Part print with two shaded views. Sizes in mm from the minimum x, y, z corner. Round coordinates to 2 decimals unless told otherwise and drop trailing zeros. Write each loop counter-clockwise with the first axis right and the second up, starting at its lowest first coordinate (ties: lowest second). Pieces come first, ordered by that corner, then holes. Notation, with made-up numbers: (2, 81) -> (57, 81) arc R22 ccw to (57, 106) -> close; hole circle Ø10 at (-23, -13). An arc over 180 degrees is marked (long way). Answer in a Markdown table with one row per item.
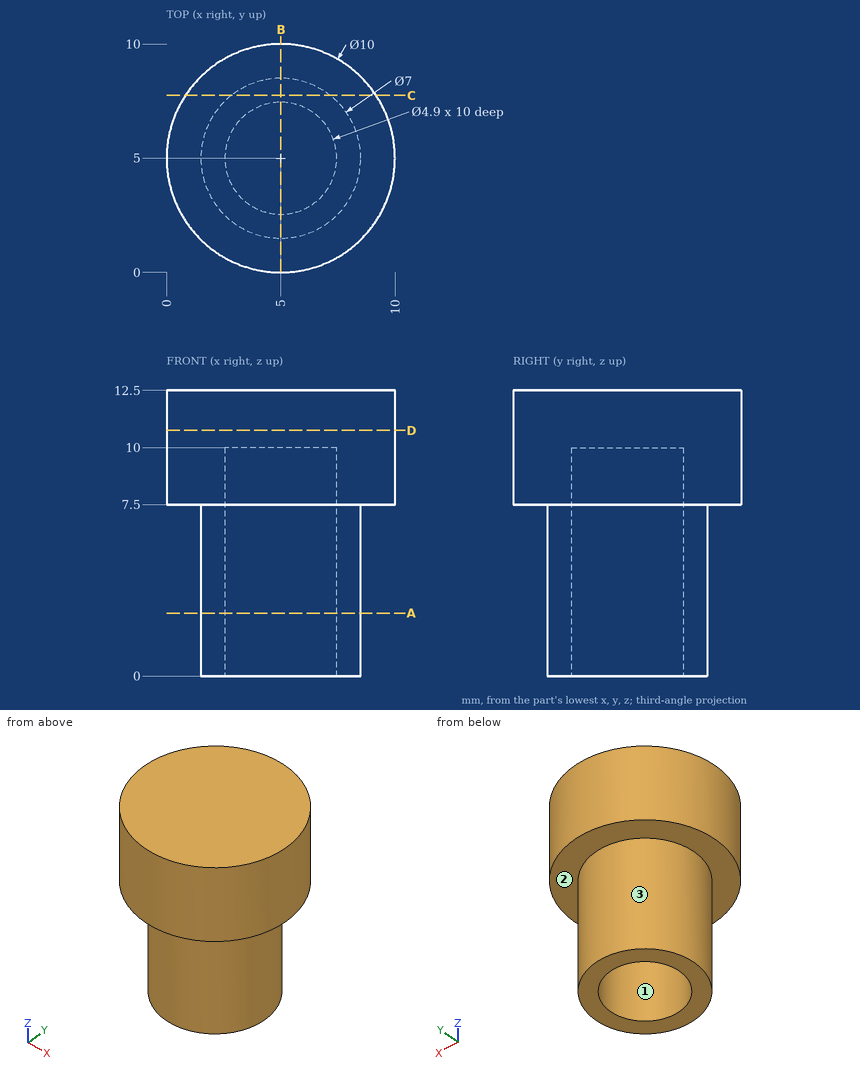
Q1. Drop flat-ended pins along their axis: P1, Ø1, axis at x = 8.5, z = 5, coming from the -Y side; P2, Ø5, axis at x = 8, z = 4, coming from the +Y side; P3, Ø2, axis at y = 4, z = 5, coming from the -X side. Give the stop position or say it passes through.
A:
| item | result |
|---|---|
| P1 | y = 3.2 |
| P2 | y = 8.46 |
| P3 | x = 1.5 |
Q2. Two-plate mould, pull along Y, no slides. Class the marked faces 1, 2 and 3: released by +Y, released by -Y, zero draft, split by the parting line, or undercut.
A:
| item | result |
|---|---|
| face 1 | undercut |
| face 2 | zero draft |
| face 3 | split by the parting line |
Q3. Saw through at D-D on z = 10.75. Write the cut outline in (x, y).
A:
| item | result |
|---|---|
| outline | circle Ø10 at (5, 5) |
Q4. Saw through at C-C on y = 7.75. Write the cut outline in (x, z).
A:
| item | result |
|---|---|
| outline | (0.82, 7.5) -> (2.83, 7.5) -> (2.83, 0) -> (7.17, 0) -> (7.17, 7.5) -> (9.18, 7.5) -> (9.18, 12.5) -> (0.82, 12.5) -> close |
Q5. Saw through at A-A on z = 2.75. Write the cut outline in (x, y), plus the area to 3 significant figures.
A:
| item | result |
|---|---|
| outline | circle Ø7 at (5, 5); hole circle Ø4.9 at (5, 5) |
| area | 19.6 mm² |
Q6. Wall check: line 1 (Y direction, x = 5, z = 7); line 2 (Y direction, x = 5, z = 7.75); line 3 (Z direction, x = 9.25, y = 5.5). Give the ranges that are in metal, low to high. Write a range as [from, to].
A:
| item | result |
|---|---|
| line 1 | [1.5, 2.55], [7.45, 8.5] |
| line 2 | [0, 2.55], [7.45, 10] |
| line 3 | [7.5, 12.5] |
Q7. Saw through at B-B on x = 5. Write the cut outline in (y, z), plus the area to 3 significant figures.
A:
| item | result |
|---|---|
| outline | (0, 7.5) -> (1.5, 7.5) -> (1.5, 0) -> (2.55, 0) -> (2.55, 10) -> (7.45, 10) -> (7.45, 0) -> (8.5, 0) -> (8.5, 7.5) -> (10, 7.5) -> (10, 12.5) -> (0, 12.5) -> close |
| area | 53.5 mm² |
